Model file for the job. Use its own axes, mm. A direction names the side the tool comes from. Coordinates: 2 decimals unless noted, no trailing zeros. Write each loop counter-clockwise with the first axis right and the second up, starting at its lowest first coordinate (ties: lowest second). Pieces come first, ordered by that corner, then holes. Notation, with made-up numbers: (56, 83.25) -> (112, 83.25) arc R8 ccw to (112, 98.25) -> close; hole circle Ø2 at (-10.5, -30.75). An arc over 180 degrees is marked (long way). Write item = value, one per line. Start each with the question number.
from build123d import *

# Parameters (mm, degrees)
SKETCH_1_W          = 30
SKETCH_1_H          = 27
EXTRUDE_1_DEPTH     = 4
SKETCH_2_W          = 4
SKETCH_2_H          = 27
EXTRUDE_2_DEPTH     = 26
CUT_EXTRUDE_1_DEPTH = 37


with BuildPart() as part:
    # 草图1 → 凸台-拉伸1 (new body)
    with BuildSketch(Plane.XY):
        with Locations((15, 13.5)):
            Rectangle(SKETCH_1_W, SKETCH_1_H)
        with BuildLine():
            Line((8.5, 17), (18.5, 17))
            ThreePointArc((18.5, 17), (22, 13.5), (18.5, 10))
            Line((18.5, 10), (8.5, 10))
            ThreePointArc((8.5, 10), (5, 13.5), (8.5, 17))
        make_face(mode=Mode.SUBTRACT)
    extrude(amount=EXTRUDE_1_DEPTH)

    # 草图2 → 凸台-拉伸2 (add)
    with BuildSketch(Plane.XY.offset(4)):
        with Locations((28, 13.5)):
            Rectangle(SKETCH_2_W, SKETCH_2_H)
    extrude(amount=EXTRUDE_2_DEPTH)

    # 草图3 → 切除-拉伸1 (cut)
    with BuildSketch(Plane.ZY.offset(-26)):
        with BuildLine():
            Line((21.5, 10), (11.5, 10))
            ThreePointArc((11.5, 10), (8, 13.5), (11.5, 17))
            Line((11.5, 17), (21.5, 17))
            ThreePointArc((21.5, 17), (25, 13.5), (21.5, 10))
        make_face()
    extrude(amount=-CUT_EXTRUDE_1_DEPTH, mode=Mode.SUBTRACT)


solid = part.part
(1) Drill centre lines: line 1 along Y through (x, z) = (11, 1.75); line 2 along X through (y, z) = (15.5, 6.25); line 3 along Z through (x, y) = (24.75, 2.75). Where is each one in solid material? Low to high.
(2) Drop flat-ended pins along their axis: pin 1 Ø6 at (x, y) = (7.5, 17) entering from +Z; pin 2 Ø13 at (y, z) = (8.5, 20.5) entering from -X. Give the stop position or say it passes through.
(3) Saw through at B-B (z = 13.25). Give the cut face in (x, y).
(4) Saw through at C-C (z = 3.25). Give the cut face in (x, y), then the cut area to 3 significant figures.
(5) 3-axis set-ups, long thin cutter, end or side, ignore diameter. For faces 4 (the face through (13, 20, 4)), 5 (the face through (14, 10, 2)), 6 (the face through (28, 17, 16)): which of +Z, -Z, +X, -X, +Y, -Y reach the whole face in a straight line?
(6) Saw through at D-D (y = 15.5). Give the cut face in (x, z).
(7) Mould opens along Y. For faces 1 (the face through (21.6, 0, 3.8)), 2 (the face through (5, 13.4, 2)), 3 (the face through (0, 13, 2)) say: released by +Y, released by -Y, zero draft, split by the parting line, or undercut.
(8) Saw through at A-A (x = 10). Give the cut face in (y, z), then the cut area to 3 significant figures.
Returned:
q1.line_1 = 0 to 10, 17 to 27
q1.line_2 = 26 to 30
q1.line_3 = 0 to 4
q2.pin_1 = 4
q2.pin_2 = 26
q3.outline = (26, 0) -> (30, 0) -> (30, 10) -> (26, 10) -> close; (26, 17) -> (30, 17) -> (30, 27) -> (26, 27) -> close
q4.outline = (0, 0) -> (30, 0) -> (30, 27) -> (0, 27) -> close; hole (8.5, 10) -> (18.5, 10) arc R3.5 ccw to (18.5, 17) -> (8.5, 17) arc R3.5 ccw to start
q4.area = 702 mm2
q5.face_4 = +Z, -X, +Y, -Y
q5.face_5 = +Z, -Z
q5.face_6 = +X, -X
q6.outline = (0, 0) -> (5.63, 0) -> (5.63, 4) -> (0, 4) -> close; (21.37, 0) -> (30, 0) -> (30, 8.63) -> (26, 8.63) -> (26, 4) -> (21.37, 4) -> close; (26, 24.37) -> (30, 24.37) -> (30, 30) -> (26, 30) -> close
q7.face_1 = released by -Y
q7.face_2 = undercut
q7.face_3 = zero draft
q8.outline = (0, 0) -> (10, 0) -> (10, 4) -> (0, 4) -> close; (17, 0) -> (27, 0) -> (27, 4) -> (17, 4) -> close
q8.area = 80.0 mm2
